from build123d import *

# Parameters (mm, degrees)
EXTRUDE_1_DEPTH     = 25
EXTRUDE_2_DEPTH     = 2
CUT_EXTRUDE_1_REACH = 87
SKETCH_4_R          = 2.1
CUT_EXTRUDE_2_REACH = 87
FILLET_1_R          = 5
EXTRUDE_3_DEPTH     = 2
SKETCH_7_R          = 7.5
CUT_EXTRUDE_3_DEPTH = 51


with BuildPart() as part:
    # 草图1 → 凸台-拉伸1 (new body, symmetric)
    with BuildSketch(Plane(origin=(0, 0, 0), x_dir=(0, 0, -1), z_dir=(1, 0, 0))):
        Polygon((0, 0), (0, 85), (30, 85), (30, 82), (3, 82), (3, 3), (83, 3), (83, 0), align=None)
    extrude(amount=EXTRUDE_1_DEPTH, both=True)

    # 草图2 → 凸台-拉伸2 (add)
    with BuildSketch(Plane(origin=(25, 0, 0), x_dir=(0, 0, -1), z_dir=(1, 0, 0))):
        Polygon((43, 3), (3, 3), (3, 82), (18, 82), align=None)
    extrude(amount=-EXTRUDE_2_DEPTH)

    # 草图4 → 切除-拉伸1 (cut, up to next)
    with BuildSketch(Plane(origin=(0, 85, 0), x_dir=(1, 0, 0), z_dir=(0, 1, 0)), mode=Mode.PRIVATE) as cut_extrude_1_sk1:
        with Locations((-17, 26)):
            Circle(SKETCH_4_R)
    cut_extrude_1_tool1 = extrude(cut_extrude_1_sk1.sketch, amount=-CUT_EXTRUDE_1_REACH, mode=Mode.PRIVATE) & part.part
    add(cut_extrude_1_tool1.solids().sort_by_distance((-17, 85, -26))[0], mode=Mode.SUBTRACT)
    # 草图4 → 切除-拉伸1 (cut, up to next)
    with BuildSketch(Plane(origin=(0, 85, 0), x_dir=(1, 0, 0), z_dir=(0, 1, 0)), mode=Mode.PRIVATE) as cut_extrude_1_sk2:
        with Locations((-17, 8)):
            Circle(SKETCH_4_R)
    cut_extrude_1_tool2 = extrude(cut_extrude_1_sk2.sketch, amount=-CUT_EXTRUDE_1_REACH, mode=Mode.PRIVATE) & part.part
    add(cut_extrude_1_tool2.solids().sort_by_distance((-17, 85, -8))[0], mode=Mode.SUBTRACT)
    # 草图4 → 切除-拉伸1 (cut, up to next)
    with BuildSketch(Plane(origin=(0, 85, 0), x_dir=(1, 0, 0), z_dir=(0, 1, 0)), mode=Mode.PRIVATE) as cut_extrude_1_sk3:
        with Locations((17, 8)):
            Circle(SKETCH_4_R)
    cut_extrude_1_tool3 = extrude(cut_extrude_1_sk3.sketch, amount=-CUT_EXTRUDE_1_REACH, mode=Mode.PRIVATE) & part.part
    add(cut_extrude_1_tool3.solids().sort_by_distance((17, 85, -8))[0], mode=Mode.SUBTRACT)
    # 草图4 → 切除-拉伸1 (cut, up to next)
    with BuildSketch(Plane(origin=(0, 85, 0), x_dir=(1, 0, 0), z_dir=(0, 1, 0)), mode=Mode.PRIVATE) as cut_extrude_1_sk4:
        with Locations((17, 26)):
            Circle(SKETCH_4_R)
    cut_extrude_1_tool4 = extrude(cut_extrude_1_sk4.sketch, amount=-CUT_EXTRUDE_1_REACH, mode=Mode.PRIVATE) & part.part
    add(cut_extrude_1_tool4.solids().sort_by_distance((17, 85, -26))[0], mode=Mode.SUBTRACT)

    # 草图5 → 切除-拉伸2 (cut, up to next)
    with BuildSketch(Plane.XZ, mode=Mode.PRIVATE) as cut_extrude_2_sk1:
        with BuildLine():
            Line((-12.9, -11), (-12.9, -31))
            ThreePointArc((-12.9, -31), (-15, -33.1), (-17.1, -31))
            Line((-17.1, -31), (-17.1, -11))
            ThreePointArc((-17.1, -11), (-15, -8.9), (-12.9, -11))
        make_face()
    cut_extrude_2_tool1 = extrude(cut_extrude_2_sk1.sketch, amount=-CUT_EXTRUDE_2_REACH, mode=Mode.PRIVATE) & part.part
    add(cut_extrude_2_tool1.solids().sort_by_distance((-15, 0, -21))[0], mode=Mode.SUBTRACT)
    # 草图5 → 切除-拉伸2 (cut, up to next)
    with BuildSketch(Plane.XZ, mode=Mode.PRIVATE) as cut_extrude_2_sk2:
        with BuildLine():
            Line((-12.9, -51), (-12.9, -71))
            ThreePointArc((-12.9, -71), (-15, -73.1), (-17.1, -71))
            Line((-17.1, -71), (-17.1, -51))
            ThreePointArc((-17.1, -51), (-15, -48.9), (-12.9, -51))
        make_face()
    cut_extrude_2_tool2 = extrude(cut_extrude_2_sk2.sketch, amount=-CUT_EXTRUDE_2_REACH, mode=Mode.PRIVATE) & part.part
    add(cut_extrude_2_tool2.solids().sort_by_distance((-15, 0, -61))[0], mode=Mode.SUBTRACT)
    # 草图5 → 切除-拉伸2 (cut, up to next)
    with BuildSketch(Plane.XZ, mode=Mode.PRIVATE) as cut_extrude_2_sk3:
        with BuildLine():
            Line((12.9, -51), (12.9, -71))
            ThreePointArc((12.9, -71), (15, -73.1), (17.1, -71))
            Line((17.1, -71), (17.1, -51))
            ThreePointArc((17.1, -51), (15, -48.9), (12.9, -51))
        make_face()
    cut_extrude_2_tool3 = extrude(cut_extrude_2_sk3.sketch, amount=-CUT_EXTRUDE_2_REACH, mode=Mode.PRIVATE) & part.part
    add(cut_extrude_2_tool3.solids().sort_by_distance((15, 0, -61))[0], mode=Mode.SUBTRACT)
    # 草图5 → 切除-拉伸2 (cut, up to next)
    with BuildSketch(Plane.XZ, mode=Mode.PRIVATE) as cut_extrude_2_sk4:
        with BuildLine():
            Line((12.9, -11), (12.9, -31))
            ThreePointArc((12.9, -31), (15, -33.1), (17.1, -31))
            Line((17.1, -31), (17.1, -11))
            ThreePointArc((17.1, -11), (15, -8.9), (12.9, -11))
        make_face()
    cut_extrude_2_tool4 = extrude(cut_extrude_2_sk4.sketch, amount=-CUT_EXTRUDE_2_REACH, mode=Mode.PRIVATE) & part.part
    add(cut_extrude_2_tool4.solids().sort_by_distance((15, 0, -21))[0], mode=Mode.SUBTRACT)

    # 圆角1
    fillet_1_edges = [part.edges().sort_by_distance(p)[0] for p in [
        (-25, 1.5, -83),
        (25, 1.5, -83),
    ]]
    fillet(fillet_1_edges, radius=FILLET_1_R)

    # 草图6 → 凸台-拉伸3 (add)
    with BuildSketch(Plane.ZY.offset(25)):
        Polygon((-43, 3), (-3, 3), (-3, 82), (-18, 82), align=None)
    extrude(amount=-EXTRUDE_3_DEPTH)

    # 草图7 → 切除-拉伸3 (cut, through all)
    with BuildSketch(Plane(origin=(25, 0, 0), x_dir=(0, 0, -1), z_dir=(1, 0, 0))):
        with Locations((15, 30)):
            Circle(SKETCH_7_R)
    extrude(amount=-CUT_EXTRUDE_3_DEPTH, mode=Mode.SUBTRACT)


solid = part.part
The listing builds one solid part. Answer for the finished solid, in the listing's coordinates (mm). A direction names the side the tool comes from. Give positions to 0.01 mm unless a question says otherwise; leave off trailing zeros. Write each loop counter-clockwise with the first axis right and the second up, starting at its lowest first coordinate (ties: lowest second). Pieces come first, ordered by that corner, then holes.
Item 1: Determine the mould class of faces 6 (the cylindrical face through (18.13, 83.52, -27.77)), 7 (the flat face through (25, 36, -22)), 8 (the flat face through (0, 2, -83)) for opening direction X: released by +X, released by -X, zero draft, split by the parting line, or undercut.
Item 2: Section C-C, the plane z = -41.5 is taken. Write down the section's boundary in (x, y).
Item 3: Section D-D, the plane x = -5 is taken. Write down the section's boundary in (y, z).
Item 4: Find the intervals of material crossed by line 1 along Z through (x, y) = (17, 84.1); line 2 along X through (y, z) = (83, -8); line 3 along Y through (x, z) = (-3.5, -27), in increasing order.
Item 5: Section A-A, the plane z = -26 is taken. Write down the section's boundary in (x, y), plus the area to 3 significant figures.
Item 6: Flat-ended cylindrical pins translate along their axes: P1, Ø5, axis at y = 55, z = -27, coming from the +X side; P2, Ø23, axis at x = 5.5, y = 36.5, coming from the -Z side; P3, Ø4, axis at x = 18.5, z = -47.5, coming from the +Y side; P4, Ø3.5, axis at x = -5, y = 83, coming from the -Z side. Find the tip coordinate at first contact, or state that the pin passes through.
Item 7: Section B-B, the plane y = 33.5 is taken. Write down the section's boundary in (x, z), plus the area to 3 significant figures.
Item 8: Which of the six approach directions +Z, -Z, +X, -X, +Y, -Y give full straight-line access (tool end or side, diameter ignored) to faces 1 (the cylindrical face through (15, 1.5, -33.1)), 2 (the cylindrical face through (15, 1.5, -8.9)), 3 (the flat face through (0, 3, -42)), 4 (the flat face through (0, 84, -30)), 5 (the flat face through (24.014, 43.053, -30.325))?
Completed:
1. face 6: undercut
1. face 7: released by +X
1. face 8: zero draft
2. outline: (-25, 0) - (25, 0) - (25, 7.74) - (23, 7.74) - (23, 3) - (-23, 3) - (-23, 7.74) - (-25, 7.74) - close
3. outline: (0, -83) - (3, -83) - (3, -3) - (82, -3) - (82, -30) - (85, -30) - (85, 0) - (0, 0) - close
4. line 1: z = -30 to -28.1, -23.9 to -10.1, -5.9 to 0
4. line 2: x = -25 to -19.1, -14.9 to 14.9, 19.1 to 25
4. line 3: y = 0 to 3, 82 to 85
5. outline: (-25, 0) - (-17.1, 0) - (-17.1, 3) - (-23, 3) - (-23, 56.72) - (-25, 56.72) - close; (-25, 82) - (-19.1, 82) - (-19.1, 85) - (-25, 85) - close; (-14.9, 82) - (14.9, 82) - (14.9, 85) - (-14.9, 85) - close; (-12.9, 0) - (12.9, 0) - (12.9, 3) - (-12.9, 3) - close; (17.1, 0) - (25, 0) - (25, 56.72) - (23, 56.72) - (23, 3) - (17.1, 3) - close; (19.1, 82) - (25, 82) - (25, 85) - (19.1, 85) - close
5. area: 464 mm2
6. P1: stops at x = 25
6. P2: stops at z = -3
6. P3: stops at y = 3
6. P4: stops at z = -30
7. outline: (-25, -33.35) - (-23, -33.35) - (-23, -21.63) - (-25, -21.63) - close; (-25, -8.37) - (-23, -8.37) - (-23, -3) - (23, -3) - (23, -8.37) - (25, -8.37) - (25, 0) - (-25, 0) - close; (23, -33.35) - (25, -33.35) - (25, -21.63) - (23, -21.63) - close
7. area: 218 mm2
8. face 1: +Y, -Y
8. face 2: -Y
8. face 3: -Z
8. face 4: -Z, +X, -X, +Y
8. face 5: -Z, +X, -X
